```python
from build123d import *

# Parameters (mm, degrees)
F1_DEPTH = 12.7
F3_DEPTH = 12.7


with BuildPart() as f1:
    # F0 (on Right) → F1 (new body)
    with BuildSketch(Plane.YZ):
        with BuildLine():
            Line((-254, 30.48), (-177.8, 30.48))
            Line((-177.8, 30.48), (-177.8, 36.651972))
            ThreePointArc((-177.8, 36.651972), (-179.659872, 41.1421), (-184.15, 43.001972))
            Line((-184.15, 43.001972), (-226.105012, 43.001972))
            ThreePointArc((-226.105012, 43.001972), (-231.264992, 45.651011), (-232.119778, 51.387921))
            Line((-232.119778, 51.387921), (-216.562416, 97.348726))
            Line((-216.562416, 97.348726), (-229.917262, 103.920899))
            Line((-229.917262, 103.920899), (-233.404353, 96.835028))
            Line((-233.404353, 96.835028), (-231.125369, 95.713497))
            Line((-231.125369, 95.713497), (-228.779319, 100.480739))
            Line((-228.779319, 100.480739), (-221.144723, 96.723609))
            Line((-221.144723, 96.723609), (-251.986832, 34.051552))
            Line((-251.986832, 34.051552), (-259.914278, 37.22636))
            Line((-259.914278, 37.22636), (-259.914278, 43.183118))
            Line((-259.914278, 43.183118), (-263.23086, 43.274231))
            Line((-263.23086, 43.274231), (-263.23086, 34.176804))
            Line((-263.23086, 34.176804), (-254, 30.48))
        make_face()
    extrude(amount=F1_DEPTH)

    # F2 (on face) → F3 (join)
    with BuildSketch(Plane.YZ.offset(12.7)):
        with BuildLine():
            Line((-247.65, 30.48), (-254, 30.48))
            Line((-254, 30.48), (-254, 18.415))
            ThreePointArc((-254, 18.415), (-253.070064, 16.169936), (-250.825, 15.24))
            ThreePointArc((-250.825, 15.24), (-248.579936, 16.169936), (-247.65, 18.415))
            Line((-247.65, 18.415), (-247.65, 30.48))
        make_face()
    extrude(amount=-F3_DEPTH)


solid = f1.part
```
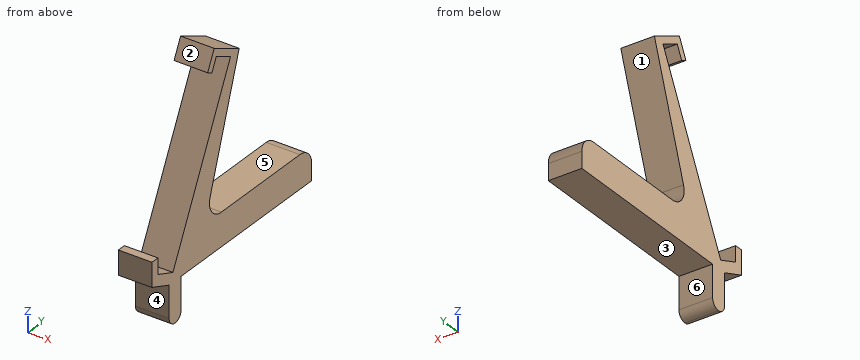
The model under review builds one solid part; all positions refer to its coordinate system, in mm. Face numbers are marked on the shaded views. A direction names the side the tool comes from. Coordinates: 2 decimals unless noted, no trailing zeros. Write each loop counter-clockwise with the first axis right and the second up, starting at its lowest first coordinate (ties: lowest second). Pieces come first, ordered by that corner, then holes.
1) Clearance check with flat-ended pins moving along their axes: pin 1 Ø2 at (x, y) = (10, -249.5) entering from -Z; pin 2 Ø6.5 at (x, y) = (9.5, -201.5) entering from +Z; pin 3 Ø1.8 at (x, z) = (6, 40.5) entering from +Y. State where each tip first meets the part, or that it passes through.
2) We need section D-D on y = -202. State the section outline as (x, z) points.
3) We need section C-C on z = 23. State the section outline as (x, y) points, then the cut area to 3 significant figures.
4) Machinability: for the marked faces 4, 5 and 6, which of the approach directions +Z, -Z, +X, -X, +Y, -Y give a long, thin tool a straight path to every point of the face, cutting with its end or side? Answer none if there is none.
5) We need section B-B on z = 41.5. State the section outline as (x, y) points, then the cut area to 3 significant figures.
6) The part is to be moulded in two halves that separate along Z. For the marked faces 1, 2 and 3, say which applies: pulls with the +Z half, pulls with the -Z half, needs draft (parallel to the pull), parting line crosses it, or undercut.
7) To check wall thickness, follow probe 1 along Z at (x, y) = (3.25, -208); probe 2 along Y at (x, z) = (5, 19.5); probe 3 along Y at (x, z) = (3.5, 96). State the ranges of each line that lie inside material, in increasing order.
Answer list:
1. pin 1: stops at z = 15.26
1. pin 2: stops at z = 43
1. pin 3: stops at y = -178.53
2. outline: (0, 30.48) - (12.7, 30.48) - (12.7, 43) - (0, 43) - close
3. outline: (0, -254) - (12.7, -254) - (12.7, -247.65) - (0, -247.65) - close
3. area: 80.6 mm2
4. face 4: -Z, +X, -X, -Y
4. face 5: +X, -X, +Y
4. face 6: -Z, +X, -X, +Y
5. outline: (0, -263.23) - (12.7, -263.23) - (12.7, -259.91) - (0, -259.91) - close; (0, -248.32) - (12.7, -248.32) - (12.7, -180.05) - (0, -180.05) - close
5. area: 909 mm2
6. face 1: undercut
6. face 2: pulls with the +Z half
6. face 3: pulls with the -Z half
7. probe 1: z = 30.48 to 43
7. probe 2: y = -254 to -247.65
7. probe 3: y = -231.71 to -230.98, -221.5 to -217.02
